Design review of the part built by this model. Coordinates are the model's own, in mm. Face numbers are marked on the shaded views. A direction names the side the tool comes from. Round coordinates to 2 decimals unless told otherwise and drop trailing zeros. Write each loop counter-clockwise with the first axis right and the second up, starting at its lowest first coordinate (ties: lowest second). Pieces come first, ordered by that corner, then holes. Notation, with made-up numbers: M -18,2 L 30,2 A17 cw 30,11 Z; hole C -27,-18 d1. An arc over 180 degrees is marked long. Use CSV: the item, a comma, the result in double quotes.
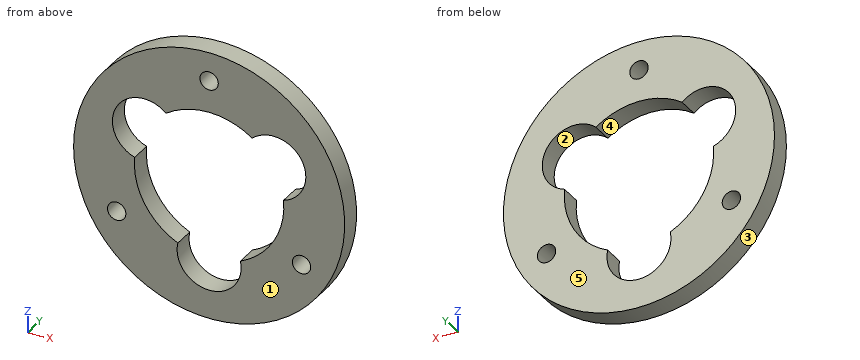
Autodesk Inventor part; units mm, degrees
ref_plane "YZ Plane" through (0, 0, 0) normal (1, 0, 0) x (0, 1, 0)
ref_plane "XZ Plane" through (0, 0, 0) normal (0, 1, 0) x (-1, 0, 0)
ref_plane "XY Plane" through (0, 0, 0) normal (0, 0, 1) x (1, 0, 0)
sketch "スケッチ1" plane through (0, 0, 0) normal (0, 1, 0) x (-1, 0, 0)
  circle A0 centre (0, 0) radius 31.75
  dimension "d0" = 63.5
extrude "押し出し1" add sketch "スケッチ1" along normal blind 5
sketch "スケッチ4" plane through (0, 5, 0) normal (0, 1, 0) x (1, 0, 0)
  circle A0 centre (0, 0) radius 17.5
  dimension "d9" = 35
extrude "押し出し4" cut sketch "スケッチ4" against normal through all
sketch "スケッチ5" plane through (0, 5, 0) normal (0, 1, 0) x (1, 0, 0)
  circle A0 centre (0, 0) radius 17.5
  circle A1 centre (0, 17.5) radius 7.5
  circle A2 centre (-15.1554, -8.75) radius 7.5
  circle A3 centre (15.1554, -8.75) radius 7.5
  point P0 (7.3258, 15.8929)
  point P1 (-7.3258, 15.8929)
  point P2 (-10.1007, -14.2907)
  point P3 (-17.4265, -1.6021)
  point P4 (10.1007, -14.2907)
  point P5 (17.4265, -1.6021)
  dimension "d12" = 15
  dimension "d30" = 360
extrude "押し出し5" cut sketch "スケッチ5" against normal through all contours A0 A1 | A3 A0 | A0 A2 picked at (-2.636, 19.4451) picked at (15.4225, -12.052) picked at (-18.1566, -7.4199)
sketch "スケッチ6" plane through (0, 5, 0) normal (0, 1, 0) x (1, 0, 0)
  circle A0 centre (0, 0) radius 25 construction
  circle A1 centre (21.6506, 12.5) radius 2.15
  line L0 (0, 0) -> (21.6506, 12.5) construction
  line L1 (0, 0) -> (35.9214, 0) construction
  circle A2 centre (-21.6506, 12.5) radius 2.15
  circle A3 centre (0, -25) radius 2.15
  dimension "d19" = 50
  dimension "d20" = 4.3
  dimension "d21" = 30
  dimension "d24" = 360
extrude "押し出し6" cut sketch "スケッチ6" against normal through all
properties part number "B_probe_bearing" material "PAEK 樹脂"
1) Add section A-A on z = 0. Write out the cut boundary in (x, y), then the cut area to 4 significant figures.
Answers:
outline,"M -31.75,0 L -17.5,0 L -17.5,5 L -31.75,5 Z; M 17.5,0 L 31.75,0 L 31.75,5 L 17.5,5 Z"
area,"142.5 mm²"
2) Add section D-D on x = 13. Write out the cut boundary in (y, z).
Answers:
outline,"M 0,-28.97 L 5,-28.97 L 5,-11.72 L 0,-11.72 Z; M 0,15.93 L 5,15.93 L 5,28.97 L 0,28.97 Z"
3) The part is to be moulded in two halves that separate along Z. For the marked faces 1, 2 and 3, say which applies: released by +Z, released by -Z, zero draft, split by the parting line, or undercut.
Answers:
face 1,"zero draft"
face 2,"undercut"
face 3,"split by the parting line"
4) Machinability: for the marked faces 4 and 5, which of the approach directions +Z, -Z, +X, -X, +Y, -Y give a long, thin tool a straight path to every point of the face, cutting with its end or side? Answer none if there is none.
Answers:
face 4,"+Y, -Y"
face 5,"+Z, -Z, +X, -X, +Y"
5) For pin 1 Ø5.5 at (x, z) = (-21.65, -12.5) entering from +Y; pin 2 Ø1.5 at (y, z) = (2.5, 20.5) entering from +X; pin 3 Ø9 at (x, z) = (-15.16, 8.75) entering from +Y; pin 4 Ø1.5 at (x, y) = (18, 4) entering from +Z, all flat-tipped, find the tip position at first contact; note any pin that passes through.
Answers:
pin 1,"y = 5"
pin 2,"x = 24.86"
pin 3,"through"
pin 4,"z = 26.66"
6) Add section B-B on x = 0. Write out the cut boundary in (y, z), then the cut area to 3 significant figures.
Answers:
outline,"M 0,-31.75 L 5,-31.75 L 5,-25 L 0,-25 Z; M 0,17.5 L 5,17.5 L 5,22.85 L 0,22.85 Z; M 0,27.15 L 5,27.15 L 5,31.75 L 0,31.75 Z"
area,"83.5 mm²"
7) Add section C-C on y = 1.2. Write out the cut boundary in (x, z).
Answers:
outline,"C 0,0 d63.5; hole C -21.65,-12.5 d4.3; hole M -17.43,1.6 A17.5 ccw -7.33,-15.89 A7.5 ccw long 7.33,-15.89 A17.5 ccw 17.43,1.6 A7.5 ccw long 10.1,14.29 A17.5 ccw -10.1,14.29 A7.5 ccw long Z; hole C 0,25 d4.3; hole C 21.65,-12.5 d4.3"
8) Wall thickness on line 1 along Z through (x, y) = (1.5, 0.6); line 2 along Z through (x, y) = (-1, 0.65); line 3 along X through (y, z) = (2.5, -12.5): over which ranges is each line inside the solid? List them lowest first. Write a range as [from, to].
Answers:
line 1,"[-31.71, -24.85], [17.44, 23.46], [26.54, 31.71]"
line 2,"[-31.73, -24.93], [17.47, 23.1], [26.9, 31.73]"
line 3,"[-29.19, -23.8], [-19.5, -12.25], [12.25, 19.5], [23.8, 29.19]"
